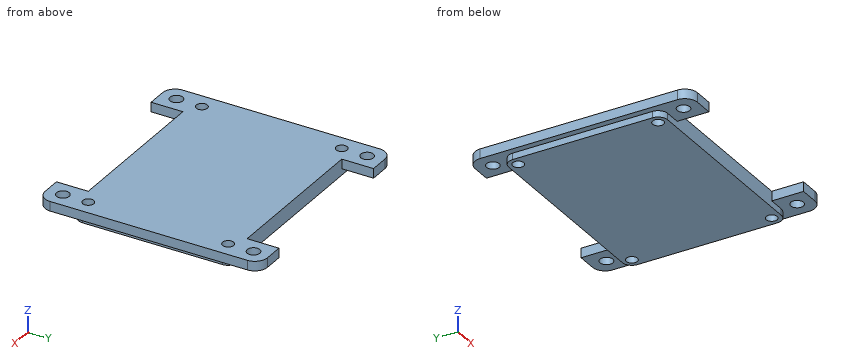
from build123d import *

# Parameters (mm, degrees)
SKETCH1_W           = 66
SKETCH1_H           = 50
SKETCH1_R           = 1.75
BOSS_EXTRUDE1_DEPTH = 2
FILLET1_R           = 3
BOSS_EXTRUDE2_START = 3
SKETCH2_R           = 1.75
SKETCH2_R_2         = 2
BOSS_EXTRUDE2_DEPTH = 3
FILLET2_R           = 4


with BuildPart() as part:
    # Sketch1 → Boss-Extrude1 (new body)
    with BuildSketch(Plane.XY):
        Rectangle(SKETCH1_W, SKETCH1_H)
        with Locations((-30, 22)):
            Circle(SKETCH1_R, mode=Mode.SUBTRACT)
        with Locations((30, 22)):
            Circle(SKETCH1_R, mode=Mode.SUBTRACT)
        with Locations(Location((30, -22, 0), (0, 0, 180))):
            Circle(SKETCH1_R, mode=Mode.SUBTRACT)
        with Locations(Location((-30, -22, 0), (0, 0, 180))):
            Circle(SKETCH1_R, mode=Mode.SUBTRACT)
    extrude(amount=BOSS_EXTRUDE1_DEPTH)

    # Fillet1
    fillet1_edges = [part.edges().sort_by_distance(p)[0] for p in [
        (33, -25, 1),
        (-33, -25, 1),
        (-33, 25, 1),
        (33, 25, 1),
    ]]
    fillet(fillet1_edges, radius=FILLET1_R)

    # Sketch2 → Boss-Extrude2 (add)
    # profile 1 of 3: a face of its own
    with BuildSketch(Plane.XY.offset(2).offset(BOSS_EXTRUDE2_START)):
        with BuildLine():
            ThreePointArc((-30, 25), (-32.121320344, 24.121320344), (-33, 22))
            Line((-33, 22), (-33, -22))
            ThreePointArc((-33, -22), (-32.121320344, -24.121320344), (-30, -25))
            Line((-30, -25), (30, -25))
            ThreePointArc((30, -25), (32.121320344, -24.121320344), (33, -22))
            Line((33, -22), (33, 22))
            ThreePointArc((33, 22), (32.121320344, 24.121320344), (30, 25))
            Line((30, 25), (-30, 25))
        make_face()
        with Locations((-30, 22)):
            Circle(SKETCH2_R, mode=Mode.SUBTRACT)
        with Locations(Location((30, -22, 0), (0, 0, 180))):
            Circle(SKETCH2_R, mode=Mode.SUBTRACT)
        with Locations(Location((-30, -22, 0), (0, 0, 180))):
            Circle(SKETCH2_R, mode=Mode.SUBTRACT)
        with Locations((30, 22)):
            Circle(SKETCH2_R, mode=Mode.SUBTRACT)
    # profile 2 of 3: a face of its own
    with BuildSketch(Plane.XY.offset(2).offset(BOSS_EXTRUDE2_START)):
        with BuildLine():
            Line((-35, 35), (-35, -35))
            Line((-35, -35), (-25, -35))
            Line((-25, -35), (-25, -25))
            Line((-25, -25), (-30, -25))
            ThreePointArc((-30, -25), (-32.121320344, -24.121320344), (-33, -22))
            Line((-33, -22), (-33, 22))
            ThreePointArc((-33, 22), (-32.121320344, 24.121320344), (-30, 25))
            Line((-30, 25), (-25, 25))
            Line((-25, 25), (-25, 35))
            Line((-25, 35), (-35, 35))
        make_face()
        with Locations((-30, -30)):
            Circle(SKETCH2_R_2, mode=Mode.SUBTRACT)
        with Locations((-30, 30)):
            Circle(SKETCH2_R_2, mode=Mode.SUBTRACT)
    # profile 3 of 3: a face of its own
    with BuildSketch(Plane.XY.offset(2).offset(BOSS_EXTRUDE2_START)):
        with BuildLine():
            Line((25, -25), (25, -35))
            Line((25, -35), (35, -35))
            Line((35, -35), (35, 35))
            Line((35, 35), (25, 35))
            Line((25, 35), (25, 25))
            Line((25, 25), (30, 25))
            ThreePointArc((30, 25), (32.121320344, 24.121320344), (33, 22))
            Line((33, 22), (33, -22))
            ThreePointArc((33, -22), (32.121320344, -24.121320344), (30, -25))
            Line((30, -25), (25, -25))
        make_face()
        with Locations((30, -30)):
            Circle(SKETCH2_R_2, mode=Mode.SUBTRACT)
        with Locations((30, 30)):
            Circle(SKETCH2_R_2, mode=Mode.SUBTRACT)
    extrude(amount=-BOSS_EXTRUDE2_DEPTH)

    # Fillet2
    fillet2_edges = [part.edges().sort_by_distance(p)[0] for p in [
        (35, -35, 3.5),
        (35, 35, 3.5),
        (-35, 35, 3.5),
        (-35, -35, 3.5),
    ]]
    fillet(fillet2_edges, radius=FILLET2_R)


solid = part.part
Here's how the part is built. I have some questions about the finished solid (model axes, mm). Round coordinates to 2 decimals unless told otherwise and drop trailing zeros. Order: outer loops, then holes, each group sorted by start corner. A loop starts at its lowest first (then second) coordinate and runs counter-clockwise, first axis right, second up. Notation, with made-up numbers: M -2.5,41.25 L 51.5,41.25 A4 ccw 51.5,45.25 Z; hole C 16.5,51 d2. An arc over 180 degrees is marked long. One line per question, with ' | ' between items.
1) Imagine slicing it at B-B, the plane z = 2.75. Count the separate pieces of the cut face and the enclosed holes in it, plus the area to 3 significant figures.
Checked values:
separate pieces: 1 | enclosed holes: 8 | area: 3,800 mm²
2) Imagine slicing it at D-D, the plane x = -22.5. Write out the boundary of the cut face in (y, z), plus the area to 3 significant figures.
Checked values:
outline: M -25,0 L 25,0 L 25,5 L -25,5 Z | area: 250 mm²
3) I need wall thicknesses on line 1 (Y direction, x = -30, z = 3.2); line 2 (X direction, y = -22, z = 3.6); line 3 (Y direction, x = -30, z = 1.65). Which ranges of each line are inside material? Lowest first, please.
Checked values:
line 1: y = -35 to -32, -28 to -23.75, -20.25 to 20.25, 23.75 to 28, 32 to 35 | line 2: x = -35 to -31.75, -28.25 to 28.25, 31.75 to 35 | line 3: y = -25 to -23.75, -20.25 to 20.25, 23.75 to 25
4) I'm going to push flat-ended pins straight in: pin 1 Ø2 at (x, y) = (-24, 16) entering from -Z; pin 2 Ø1.6 at (y, z) = (6.5, 0.5) entering from +X; pin 3 Ø0.9 at (y, z) = (-32, 3.5) entering from +X; pin 4 Ø2.5 at (x, z) = (1, 2.5) entering from +Y. Where does each tip first touch, or does it pass through?
Checked values:
pin 1: stops at z = 0 | pin 2: stops at x = 33 | pin 3: stops at x = 34.96 | pin 4: stops at y = 25
5) Imagine slicing it at C-C, the plane y = 17.5. Write out the boundary of the cut face in (x, z).
Checked values:
outline: M -35,2 L -33,2 L -33,0 L 33,0 L 33,2 L 35,2 L 35,5 L -35,5 Z
6) Imagine slicing it at A-A, the plane y = -30. Write out the boundary of the cut face in (x, z), plus the area to 3 significant figures.
Checked values:
outline: M -35,2 L -32,2 L -32,5 L -35,5 Z; M -28,2 L -25,2 L -25,5 L -28,5 Z; M 25,2 L 28,2 L 28,5 L 25,5 Z; M 32,2 L 35,2 L 35,5 L 32,5 Z | area: 36.0 mm²
